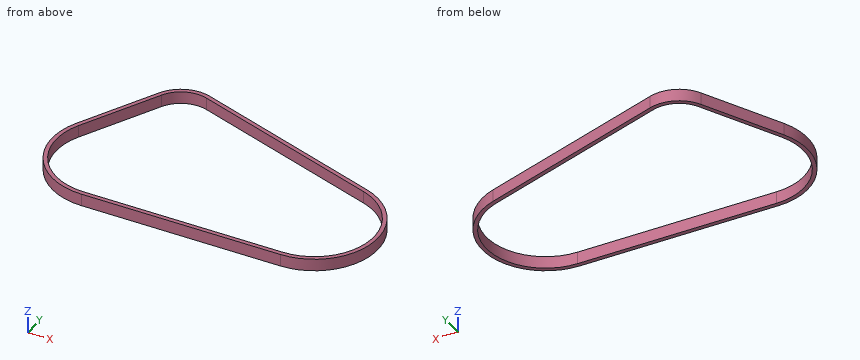
```python
from build123d import *

# Parameters (mm, degrees)
EXTRUDE_THIN1_DEPTH      = 7.5
EXTRUDE_THIN1_DEPTH_BACK = 7.5


with BuildPart() as part:
    # Sketch2 → Extrude-Thin1 (new, two sides)
    with BuildSketch(Plane.XY) as extrude_thin1_sk:
        with BuildLine():
            Line((246.24621437, -35.923587532), (13.466243252, 40.836996617))
            ThreePointArc((13.466243252, 40.836996617), (-15.71191081, 40.02668933), (-37.64999876, 20.772038739))
            Line((-37.64999876, 20.772038739), (-89.010467091, -72.320487869))
            ThreePointArc((-89.010467091, -72.320487869), (-87.882828318, -149.654747848), (-20.715120503, -188))
            Line((-20.715120503, -188), (221.819075448, -188))
            ThreePointArc((221.819075448, -188), (298.831932078, -122.370121817), (246.24621437, -35.923587532))
        make_face()
        with BuildLine():
            Line((244.680372131, -40.672075511), (11.900401013, 36.088508638))
            ThreePointArc((11.900401013, 36.088508638), (-13.884944436, 35.372423129), (-33.272091928, 18.356685397))
            Line((-33.272091928, 18.356685397), (-84.632560259, -74.735841211))
            ThreePointArc((-84.632560259, -74.735841211), (-83.577206022, -147.112776832), (-20.715120503, -183))
            Line((-20.715120503, -183), (221.819075448, -183))
            ThreePointArc((221.819075448, -183), (293.895210499, -121.57716529), (244.680372131, -40.672075511))
        make_face(mode=Mode.SUBTRACT)
    extrude(amount=EXTRUDE_THIN1_DEPTH)
    extrude(extrude_thin1_sk.sketch, amount=-EXTRUDE_THIN1_DEPTH_BACK)


solid = part.part
```
Work out the finished part from the listing and answer in its coordinate system (mm). Give positions to 0.01 mm unless a question says otherwise; leave off trailing zeros. Loops run counter-clockwise (first coordinate to the right, second up) from the corner with the lowest first, then second, coordinate; pieces in that order, holes last. Notation, with made-up numbers: M 0.5,41 L 26.5,41 A11 ccw 26.5,49 Z; hole C 48.25,75 d2. An arc over 180 degrees is marked long. One line per item, written item: value. Start each with the question number.
1. Find the intervals of material crossed by probe 1 along X at (y, z) = (-113.5, -5.5); probe 2 along Y at (x, z) = (114.5, 6); probe 3 along Y at (x, z) = (134, -3.25), in increasing order.
2. Each of these flat-tipped pins is pushed along its axis until it touches: P1, Ø8, axis at y = -5.5, z = 0, coming from the -X side; P2, Ø2, axis at x = 87.5, z = -5.5, coming from the +Y side; P3, Ø1, axis at y = -162.5, z = -1, coming from the -X side. Where does it stop, or does it pass through?
3. Find section A-A (x = 96). Give the vertices of the cut face in (y, z), and give its area (3 significant figures).
4. Find section C-C (z = -4.75). Give the vertices of the cut face in (x, y).
5. Find section B-B (y = -85). Give the vertices of the cut face in (x, z), and give its area (3 significant figures).
Reported:
1. probe 1: x = -98.64 to -93.63, 294.74 to 299.74
1. probe 2: y = -188 to -183, 2.26 to 7.52
1. probe 3: y = -188 to -183, -4.17 to 1.09
2. P1: stops at x = -54.35
2. P2: stops at y = 16.75
2. P3: stops at x = -78.85
3. outline: M -188,-7.5 L -183,-7.5 L -183,7.5 L -188,7.5 Z; M 8.36,-7.5 L 13.62,-7.5 L 13.62,7.5 L 8.36,7.5 Z
3. area: 154 mm²
4. outline: M -89.01,-72.32 A78 ccw -20.72,-188 L 221.82,-188 A78 ccw 246.25,-35.92 L 13.47,40.84 A43 ccw -37.65,20.77 Z; hole M -84.63,-74.74 A73 ccw -20.72,-183 L 221.82,-183 A73 ccw 244.68,-40.67 L 11.9,36.09 A38 ccw -33.27,18.36 Z
5. outline: M -94.6,-7.5 L -89.3,-7.5 L -89.3,7.5 L -94.6,7.5 Z; M 290.4,-7.5 L 295.7,-7.5 L 295.7,7.5 L 290.4,7.5 Z
5. area: 159 mm²
